The model under review builds one solid part; all positions refer to its coordinate system, in mm. Face numbers are marked on the shaded views. Round coordinates to 2 decimals unless told otherwise and drop trailing zeros. Order: outer loops, then holes, each group sorted by start corner. A loop starts at its lowest first (then second) coordinate and runs counter-clockwise, first axis right, second up. Notation, with made-up numbers: (14.5, 18) -> (52.5, 18) arc R25 ccw to (52.5, 30) -> close; hole circle Ø3 at (61.5, 7.5). An arc over 180 degrees is marked (long way). Use a Markdown table: item, result. Add a question column.
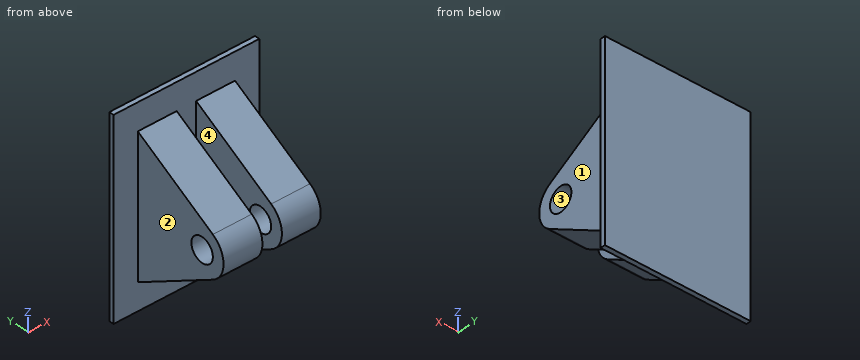
```python
from build123d import *

# Parameters (mm, degrees)
F0_W     = 76.2
F0_H     = 101.6
F1_DEPTH = 2.5
F2_R     = 6.35
F3_DEPTH = 25.4
F4_W     = 10.178574
F4_H     = 98.918622
F5_DEPTH = 75.946


with BuildPart() as f1:
    # F0 (on Front) → F1 (new body)
    with BuildSketch(Plane.XZ):
        Rectangle(F0_W, F0_H)
    extrude(amount=F1_DEPTH)

    # F2 (on Right) → F3 (join, symmetric)
    with BuildSketch(Plane.YZ):
        with BuildLine():
            Line((-46.941136, -10.998523), (0, -38.1))
            Line((0, -38.1), (0, 38.1))
            Line((0, 38.1), (-46.941136, 10.998523))
            ThreePointArc((-46.941136, 10.998523), (-53.291136, 0), (-46.941136, -10.998523))
        make_face()
        with Locations((-40.591136, 0)):
            Circle(F2_R, mode=Mode.SUBTRACT)
    extrude(amount=F3_DEPTH, both=True)

    # F4 (on Top) → F5 (cut, symmetric)
    with BuildSketch(Plane.XY):
        with Locations((0, -51.959311)):
            Rectangle(F4_W, F4_H)
    extrude(amount=F5_DEPTH, both=True, mode=Mode.SUBTRACT)


solid = f1.part
```
Q1. Add section C-C (x = -6.5). Write out the cut boundary in (y, z).
Q2. Wall thickness on line 1 (X direction, y = -16.5, z = -17.5); line 2 (Y direction, x = 20.5, z = 0); line 3 (Y direction, x = -35, z = -34.5): over which ranges is each line inside the solid? List them lowest first. Write a range as [from, to].
Q3. Add section A-A (z = 0). Write out the cut boundary in (x, y).
Q4. Add section D-D (z = -22.5). Write out the cut boundary in (x, y).
Q5. Mouldability with a two-part tool opening along X and no side actions: class the marked faces 1, 2, 3 and 4 as pulls with the +X half, pulls with the -X half, needs draft (parallel to the pull), parting line crosses it, or undercut.
Q6. Insertion check: pin 1 (2 mm diameter, centred on x = 12.5, y = -39, fed in from +Z); pin 2 (2 mm diameter, centred on x = -11, y = -9.5, fed in from -Z); pin 3 (1.5 mm diameter, centred on x = -11.5, z = -33.5, fed in from -Y); pin 4 (11.5 mm diameter, centred on y = -40.59, z = 0, fed in from -X). Each pin has a flat end and moves straight along its axis. Give the tip position at first contact, or say it passes through.
Q7. Add section B-B (y = -13.5). Write out the cut boundary in (x, z), then the cut area to 3 significant figures.
Report:
| question | item | result |
|---|---|---|
| 1 | outline | (-46.94, -11) -> (-2.5, -36.66) -> (-2.5, -50.8) -> (0, -50.8) -> (0, 50.8) -> (-2.5, 50.8) -> (-2.5, 36.66) -> (-46.94, 11) arc R12.7 ccw to start; hole circle Ø12.7 at (-40.59, 0) |
| 2 | line 1 | x = [-25.4, -5.09], [5.09, 25.4] |
| 2 | line 2 | y = [-53.29, -46.94], [-34.24, 0] |
| 2 | line 3 | y = [-2.5, 0] |
| 3 | outline | (-38.1, -2.5) -> (-25.4, -2.5) -> (-25.4, -34.24) -> (-5.09, -34.24) -> (-5.09, -2.5) -> (5.09, -2.5) -> (5.09, -34.24) -> (25.4, -34.24) -> (25.4, -2.5) -> (38.1, -2.5) -> (38.1, 0) -> (-38.1, 0) -> close; (-25.4, -53.29) -> (-5.09, -53.29) -> (-5.09, -46.94) -> (-25.4, -46.94) -> close; (5.09, -53.29) -> (25.4, -53.29) -> (25.4, -46.94) -> (5.09, -46.94) -> close |
| 4 | outline | (-38.1, -2.5) -> (-25.4, -2.5) -> (-25.4, -27.02) -> (-5.09, -27.02) -> (-5.09, -2.5) -> (5.09, -2.5) -> (5.09, -27.02) -> (25.4, -27.02) -> (25.4, -2.5) -> (38.1, -2.5) -> (38.1, 0) -> (-38.1, 0) -> close |
| 5 | face 1 | pulls with the +X half |
| 5 | face 2 | pulls with the -X half |
| 5 | face 3 | needs draft |
| 5 | face 4 | undercut |
| 6 | pin 1 | stops at z = 16.16 |
| 6 | pin 2 | stops at z = -33.19 |
| 6 | pin 3 | stops at y = -9.27 |
| 6 | pin 4 | passes through |
| 7 | outline | (-25.4, -30.31) -> (-5.09, -30.31) -> (-5.09, 30.31) -> (-25.4, 30.31) -> close; (5.09, -30.31) -> (25.4, -30.31) -> (25.4, 30.31) -> (5.09, 30.31) -> close |
| 7 | area | 2,460 mm² |
